Check sheet for the modelled part. Datum: model origin and axes. Units: mm. Face numbers are marked on the shaded views. Coordinates: 2 decimals unless noted, no trailing zeros. Write each loop counter-clockwise with the first axis right and the second up, starting at its lowest first coordinate (ties: lowest second). Pieces come first, ordered by that corner, then holes. Notation, with made-up numbers: (39.25, 79.5) -> (48.25, 79.5) arc R23 cw to (48.25, 118.5) -> close; hole circle Ø9 at (68.5, 85.25). An arc over 180 degrees is marked (long way). One line per item, written item: value. Start each with the question number.
1) Scan lines: line 1 along X through (y, z) = (323, -50.5); line 2 along Y through (x, z) = (-893, -45.5). Record each from-to range of solid material in increasing order. Write a range as [from, to].
2) Sectioned sample at A-A on y = 482. Enter the section's corners in (x, z), plus the area to 3 significant figures.
3) Gauge pin test, flat ends, axial feed: P1, Ø5, axis at x = -5, z = 3.5, coming from the -Y side; P2, Ø10, axis at x = -823, z = -62, coming from the -Y side. Record the tip position at first contact, or that the pin passes through.
4) Sectioned sample at B-B on z = -25.5. Enter the section's corners in (x, y).
5) Sectioned sample at C-C on x = -233.5. Enter the section's corners in (y, z).
6) Draft check along X on the marked faces 1, 2, 3 and 4. Enter one of: +X half, -X half, draft (parallel to the pull), parting line (faces both ways), or undercut.
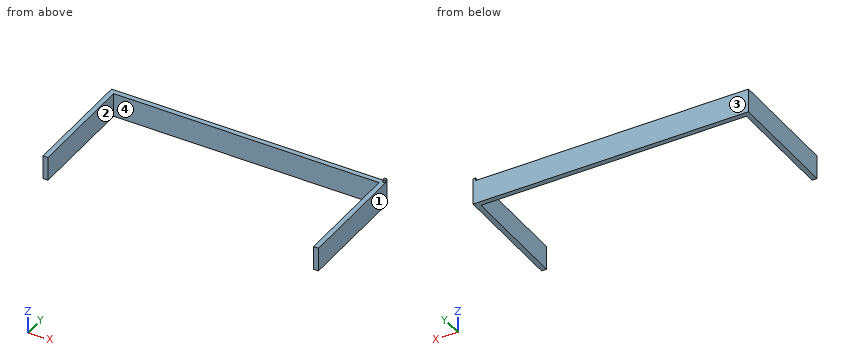
```python
from build123d import *

# Parameters (mm, degrees)
F1_DEPTH = 90
F2_W     = 10
F2_H     = 10
F3_DEPTH = 10


with BuildPart() as f1:
    # F0 (on Top) → F1 (new body)
    with BuildSketch(Plane.XY):
        Polygon((-19, 89), (0, 89), (0, 530), (-1040, 530), (-1040, 89), (-1021, 89), (-1021, 511), (-19, 511), align=None)
    extrude(amount=-F1_DEPTH)

    # F2 (on Top) → F3 (join)
    with BuildSketch(Plane.XY):
        with Locations((-5, 525)):
            Rectangle(F2_W, F2_H)
    extrude(amount=F3_DEPTH)


solid = f1.part
```
Answers:
1. line 1: x = [-1040, -1021], [-19, 0]
1. line 2: y = [511, 530]
2. outline: (-1040, -90) -> (-1021, -90) -> (-1021, 0) -> (-1040, 0) -> close; (-19, -90) -> (0, -90) -> (0, 0) -> (-19, 0) -> close
2. area: 3,420 mm2
3. P1: stops at y = 520
3. P2: stops at y = 511
4. outline: (-1040, 89) -> (-1021, 89) -> (-1021, 511) -> (-19, 511) -> (-19, 89) -> (0, 89) -> (0, 530) -> (-1040, 530) -> close
5. outline: (511, -90) -> (530, -90) -> (530, 0) -> (511, 0) -> close
6. face 1: +X half
6. face 2: undercut
6. face 3: draft
6. face 4: undercut
